Source: CAD feature listing. Evaluate the final solid. Frame: model axes, mm. Face numbers are marked on the shaded views. A direction names the side the tool comes from. Give positions to 0.01 mm unless a question says otherwise; leave off trailing zeros. Loops run counter-clockwise (first coordinate to the right, second up) from the corner with the lowest first, then second, coordinate; pieces in that order, holes last. Notation, with made-up numbers: (52.25, 75) - (90.25, 75) arc R21 cw to (90.25, 80) - close; hole circle Ø4 at (65.25, -39). An arc over 180 degrees is marked (long way). Put each result on its own line as item: value.
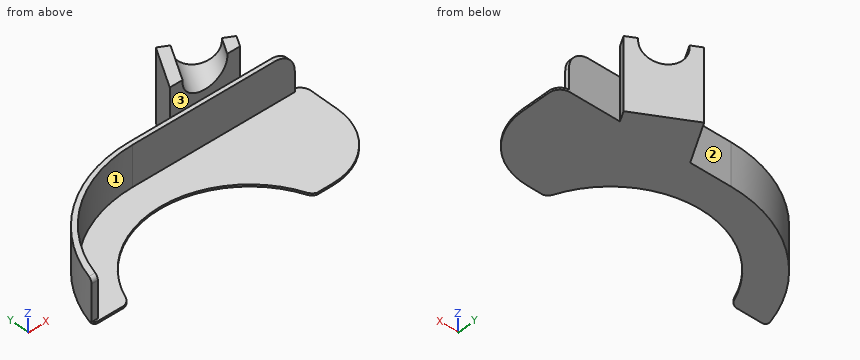
```python
from build123d import *

# Parameters (mm, degrees)
PAD_DEPTH         = 1
PAD004_DEPTH      = 20
FILLET_R          = 10
FILLET001_R       = 2
PAD005_DEPTH      = 34.5
PAD005_DEPTH_BACK = 1
SKETCH005_R       = 9.6
POCKET_DEPTH      = 107.835631986


with BuildPart() as part:
    # Sketch → Pad (new body)
    with BuildSketch(Plane.XY):
        with BuildLine():
            ThreePointArc((2.407e-07, 65), (-39.2503215588, 51.8113139915), (-62.5726380514, 17.5973))
            ThreePointArc((-62.5726380514, 17.5973), (-62.2816568518, 16.2569186959), (-61.1956, 15.4192))
            Line((-61.1956, 15.4192), (-48.0942, 15.4192))
            ThreePointArc((-48.0942, 15.4192), (-46.0175682638, 16.2684180018), (-44.5213344809, 17.9402))
            ThreePointArc((44.6290648541, 17.6705), (0.1452101265, 47.9997803539), (-44.5213344809, 17.9402))
            ThreePointArc((44.6290648541, 17.6705), (45.6957884662, 16.2979684833), (47.1679586113, 15.3736))
            Line((47.1679586113, 15.3736), (54.9232114248, 15.3841578001))
            ThreePointArc((54.9232114248, 15.3841578001), (76.1100083043, 24.1853710213), (84.8823702407, 45.38413))
            Line((84.8823702407, 59.61183), (84.8823702407, 45.38413))
            ThreePointArc((84.8823702407, 59.61183), (83.3042117859, 63.4218415452), (79.4942002407, 65))
            Line((2.407e-07, 65), (79.4942002407, 65))
        make_face()
    extrude(amount=PAD_DEPTH)

    # Sketch001 → Pad004 (new body)
    with BuildSketch(Plane.XY.offset(1)):
        with BuildLine():
            ThreePointArc((6.04881e-05, 65), (-39.6936405321, 51.4724674103), (-62.8655421025, 16.5204))
            Line((-62.8655421025, 16.5204), (-59.7655421025, 16.5204))
            ThreePointArc((6.04881e-05, 63), (-37.8013201978, 49.9422727575), (-59.7655421025, 16.5204))
            Line((80.0000604881, 63), (6.04881e-05, 63))
            Line((80.0000604881, 65), (80.0000604881, 63))
            Line((6.04881e-05, 65), (80.0000604881, 65))
        make_face()
    extrude(amount=PAD004_DEPTH)

    # Fillet
    fillet_edges = [part.edges().sort_by_distance(p)[0] for p in [
        (80.00006, 64, 21),
    ]]
    fillet(fillet_edges, radius=FILLET_R)

    # Fillet001
    fillet001_edges = [part.edges().sort_by_distance(p)[0] for p in [
        (-61.315542, 16.5204, 21),
    ]]
    fillet(fillet001_edges, radius=FILLET001_R)

    # Sketch004 → Pad005 (new body, two sides)
    with BuildSketch(Plane.XY.offset(1)) as pad005_sk:
        Polygon((31.8675134595, 85.1961524227), (57.848275573, 70.1961524227), (54.848275573, 65), (20.2072594216, 65), align=None)
    extrude(amount=PAD005_DEPTH)
    extrude(pad005_sk.sketch, amount=-PAD005_DEPTH_BACK)

    # Sketch005 → Pocket (cut, through all)
    with BuildSketch(Plane(origin=(44.8578945162, 77.6961524227, 0), x_dir=(-0.8660254038, 0.5, 0), z_dir=(0.5, 0.8660254038, 0))):
        with Locations((0, 34.5)):
            Circle(SKETCH005_R)
    extrude(amount=-POCKET_DEPTH, mode=Mode.SUBTRACT)


solid = part.part
```
1) Section query D-D, the plane x = -22.5. Output: boundary loops of the cut face in (y, z).
Check result:
outline: (42.4, 0) - (60.98, 0) - (60.98, 21) - (58.67, 21) - (58.67, 1) - (42.4, 1) - close
2) Section query A-A, the plane y = 25.5. Output: boundary loops of the cut face in (x, z), plus the area to 3 significant figures.
Check result:
outline: (-59.79, 0) - (-40.67, 0) - (-40.67, 1) - (-56.69, 1) - (-56.69, 21) - (-59.79, 21) - close; (40.67, 0) - (77.35, 0) - (77.35, 1) - (40.67, 1) - close
area: 118 mm²
3) Material intervals for line 1 along Z through (x, y) = (42.5, 23); line 2 along Y through (x, z) = (57, 5.5); line 3 along Y through (x, z) = (62, 18), sorted ascending. Write a range as [from, to].
Check result:
line 1: [0, 1]
line 2: [63, 65], [68.73, 70.69]
line 3: [63, 65]
4) Pin query (flat end, axial travel): P1, Ø4, axis at x = 11, z = 20, coming from the -Y side; P2, Ø1.5, axis at y = 26.5, z = 19, coming from the -X side; P3, Ø6.5, axis at x = 72.5, z = 13, coming from the +Y side. Return the tip coordinate at first contact, or that it passes through.
Check result:
P1: y = 63
P2: x = -59.68
P3: y = 65
5) Section query B-B, the plane z = 28. Output: boundary loops of the cut face in (x, y), plus the area to 3 significant figures.
Check result:
outline: (20.21, 65) - (29.37, 65) - (38.74, 81.23) - (31.87, 85.2) - close; (45.69, 65) - (54.85, 65) - (57.85, 70.2) - (50.98, 74.16) - close
area: 233 mm²
6) Section query C-C, the plane z = 5. Output: boundary loops of the cut face in (x, y), plus the area to 3 significant figures.
Check result:
outline: (-62.87, 16.52) - (-59.77, 16.52) arc R62 cw to (0, 63) - (80, 63) - (80, 65) - (54.85, 65) - (57.85, 70.2) - (31.87, 85.2) - (20.21, 65) - (0, 65) arc R65 ccw to start
area: 801 mm²
7) Access query for the marked faces 1, 2 and 3. Directions: +Z, -Z, +X, -X, +Y, -Y. A direction counts if a zero-diameter tool reaches every point of the face in a straight line with its end or side. Return the directions, or none.
Check result:
face 1: +Z, +X, -Y
face 2: +Z, -Z, -X, +Y
face 3: +Z, +X, -X, -Y
